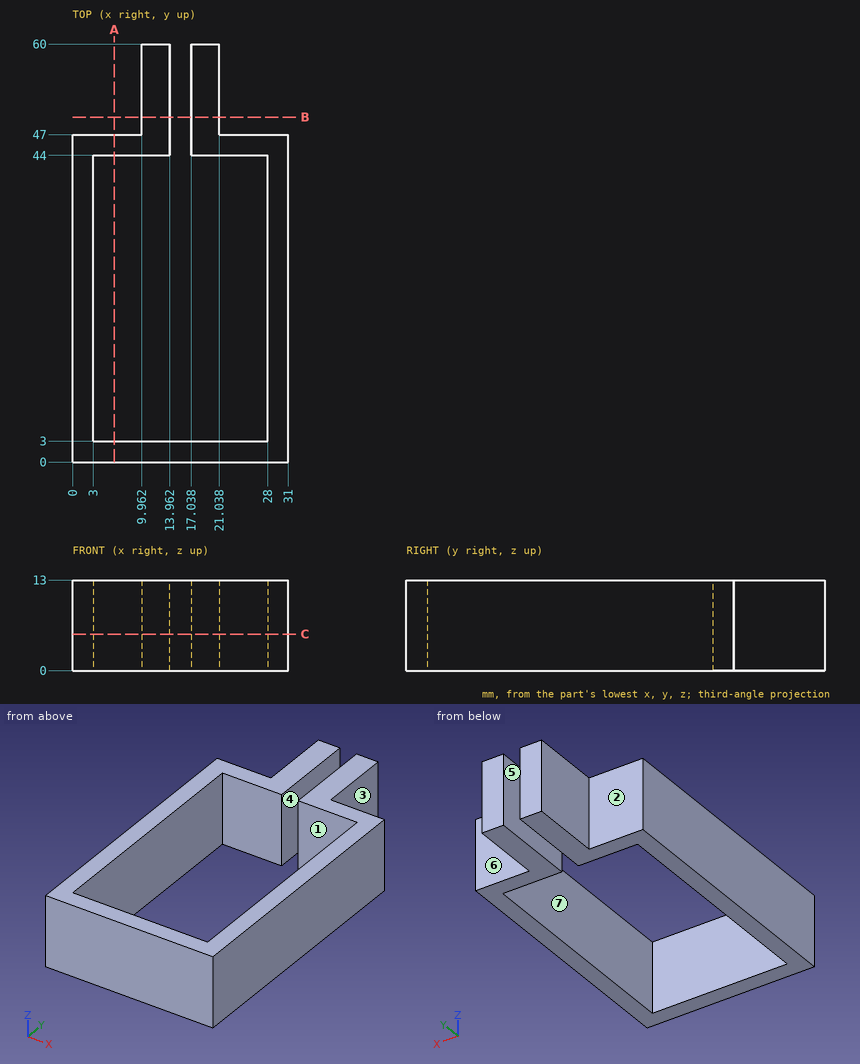
Geometry check sheet. Reference: drawing and pictorial views, mm from the part's lowest x, y, z. A direction names the side the tool comes from. Round coordinates to 2 decimals unless told otherwise and drop trailing zeros. Order: outer loops, then holes, each group sorted by start corner. A loop starts at its lowest first (then second) coordinate and runs counter-clockwise, first axis right, second up. Notation, with made-up numbers: (7, 45) - (41, 45) arc R21 ccw to (41, 83) - close; hole circle Ø9 at (25.5, 5). An arc over 180 degrees is marked (long way). Use a Markdown table: item, result. Add a question column.
1) Mould release check, pull along Y, two halves, no side actions. Record for the marked faces 5, 6 and 7: released by +Y, released by -Y, zero draft, split by the parting line, or undercut.
2) Thickness scan on line 1 along X through (y, z) = (12, 1.75); line 2 along X through (y, z) = (45.5, 6.25); line 3 along Y through (x, z) = (22, 11.25). Record the ranges inside material, lowest first.
3) Section check A-A (x = 6). Record the cut outline in (y, z).
4) Section check C-C (z = 5.25). Record the cut outline in (x, y), then the cut area to 3 significant figures.
5) Gauge pin test, flat ends, axial feed: P1, Ø4, axis at y = 49.5, z = 4, coming from the +X side; P2, Ø4, axis at y = 54, z = 7.5, coming from the -X side. Record the tip position at first contact, or that the pin passes through.
6) Section check B-B (y = 49.5). Record the cut outline in (x, z).
7) Set-up check for the marked faces 1, 2, 3 and 4: record each of +Z, -Z, +X, -X, +Y, -Y from which the full face is reachable in a straight line by a thin tool's end or side.
Established:
| question | item | result |
|---|---|---|
| 1 | face 5 | zero draft |
| 1 | face 6 | released by +Y |
| 1 | face 7 | undercut |
| 2 | line 1 | 0 to 3, 28 to 31 |
| 2 | line 2 | 0 to 13.96, 17.04 to 31 |
| 2 | line 3 | 0 to 3, 44 to 47 |
| 3 | outline | (0, 0) - (3, 0) - (3, 13) - (0, 13) - close; (44, 0) - (47, 0) - (47, 13) - (44, 13) - close |
| 4 | outline | (0, 0) - (31, 0) - (31, 47) - (21.04, 47) - (21.04, 60) - (17.04, 60) - (17.04, 44) - (28, 44) - (28, 3) - (3, 3) - (3, 44) - (13.96, 44) - (13.96, 60) - (9.96, 60) - (9.96, 47) - (0, 47) - close |
| 4 | area | 527 mm2 |
| 5 | P1 | x = 21.04 |
| 5 | P2 | x = 9.96 |
| 6 | outline | (9.96, 0) - (13.96, 0) - (13.96, 13) - (9.96, 13) - close; (17.04, 0) - (21.04, 0) - (21.04, 13) - (17.04, 13) - close |
| 7 | face 1 | +Z, -Z |
| 7 | face 2 | +Z, -Z, -X, +Y |
| 7 | face 3 | +Z, -Z, +X, +Y |
| 7 | face 4 | +Z, -Z, +Y |
